Can you work these out from the model? Positions are in its coordinate system, mm. A direction names the side the tool comes from. Give positions to 0.01 mm unless a question says otherwise; leave off trailing zeros. Write each loop counter-clockwise with the first axis right and the second up, starting at its lowest first coordinate (ties: lowest second). Pieces come first, ordered by that corner, then holes.
1. If I drill on probe 1 along X at (y, z) = (4.8, -1.65); probe 2 along Z at (x, y) = (-0.05, 3.5); probe 3 along Y at (x, z) = (2.3, -2.7), over which ranges is the centre line in solid material (lowest first)?
2. On a 3-axis mill with a long thin cutter (end or side, diameter ignored), from which of +Z, -Z, +X, -X, +Y, -Y can I reach the whole of each face in a straight line? I mean faces 1 (the flat face through (1, 4, -1)), 2 (the flat face through (0, 5, -3)), 3 (the flat face through (-1, 5, -3.2)). Say none if no direction works.
3. Suppose I cut it at C-C (z = -1.6). Please give me the cut outline in (x, y), and give its area (3 significant figures).
4. I'm going to push a flat-ended pin straight in: pin 1 (2 mm diameter, centred on x = 0.5, y = 4.5, fed in from -Z). Where does the tip first touch, or does it pass through?
5. Suppose I cut it at D-D (y = 5.55). Please give me the cut outline in (x, z), and give its area (3 significant figures).
6. Suppose I cut it at B-B (x = 0.7). Please give me the cut outline in (y, z).
7. Suppose I cut it at A-A (y = 4.35). Please give me the cut outline in (x, z).
```python
from build123d import *

# Parameters (mm, degrees)
BOSS_EXTRUDE1_DEPTH = 3
SKETCH2_W           = 3.2
SKETCH2_H           = 6
BOSS_EXTRUDE2_DEPTH = 3
BOSS_EXTRUDE3_DEPTH = 3


with BuildPart() as part:
    # Sketch1 → Boss-Extrude1 (new body)
    with BuildSketch(Plane(origin=(0, 0, 0), x_dir=(0, 0, -1), z_dir=(1, 0, 0))):
        Polygon((0, 0), (0, 3), (1.8, 4.8), (1.8, 6), (5, 0), align=None)
    extrude(amount=BOSS_EXTRUDE1_DEPTH)

    # Sketch2 → Boss-Extrude2 (add)
    with BuildSketch(Plane.ZY):
        with Locations((-1.6, 3)):
            Rectangle(SKETCH2_W, SKETCH2_H)
    extrude(amount=BOSS_EXTRUDE2_DEPTH)

    # Sketch3 → Boss-Extrude3 (add)
    with BuildSketch(Plane.ZY):
        Polygon((-5, 0), (-3.2, 0), (-3.2, 3.375), align=None)
    extrude(amount=BOSS_EXTRUDE3_DEPTH)


solid = part.part
```
Checks:
1. probe 1: x = -3 to 0
1. probe 2: z = -3.2 to 0
1. probe 3: y = 0 to 4.31
2. face 1: +Z, +X, +Y
2. face 2: -Z, +X, +Y
2. face 3: -Z, +X, -X, +Y
3. outline: (-3, 0) - (3, 0) - (3, 4.6) - (0, 4.6) - (0, 6) - (-3, 6) - close
3. area: 31.8 mm2
4. pin 1: stops at z = -3.2
5. outline: (-3, -3.2) - (0, -3.2) - (0, -2.04) - (3, -2.04) - (3, -1.8) - (0, -1.8) - (0, 0) - (-3, 0) - close
5. area: 10.3 mm2
6. outline: (0, -5) - (6, -1.8) - (4.8, -1.8) - (3, 0) - (0, 0) - close
7. outline: (-3, -3.2) - (0, -3.2) - (0, -2.68) - (3, -2.68) - (3, -1.35) - (0, -1.35) - (0, 0) - (-3, 0) - close
